The drawing under review shows one solid part. Ordinate dimensions are in mm from its lowest x, y, z. Coordinates: 2 decimals unless noted, no trailing zeros. Order: outer loops, then holes, each group sorted by start corner. A loop starts at its lowest first (then second) coordinate and runs counter-clockwise, first axis right, second up.
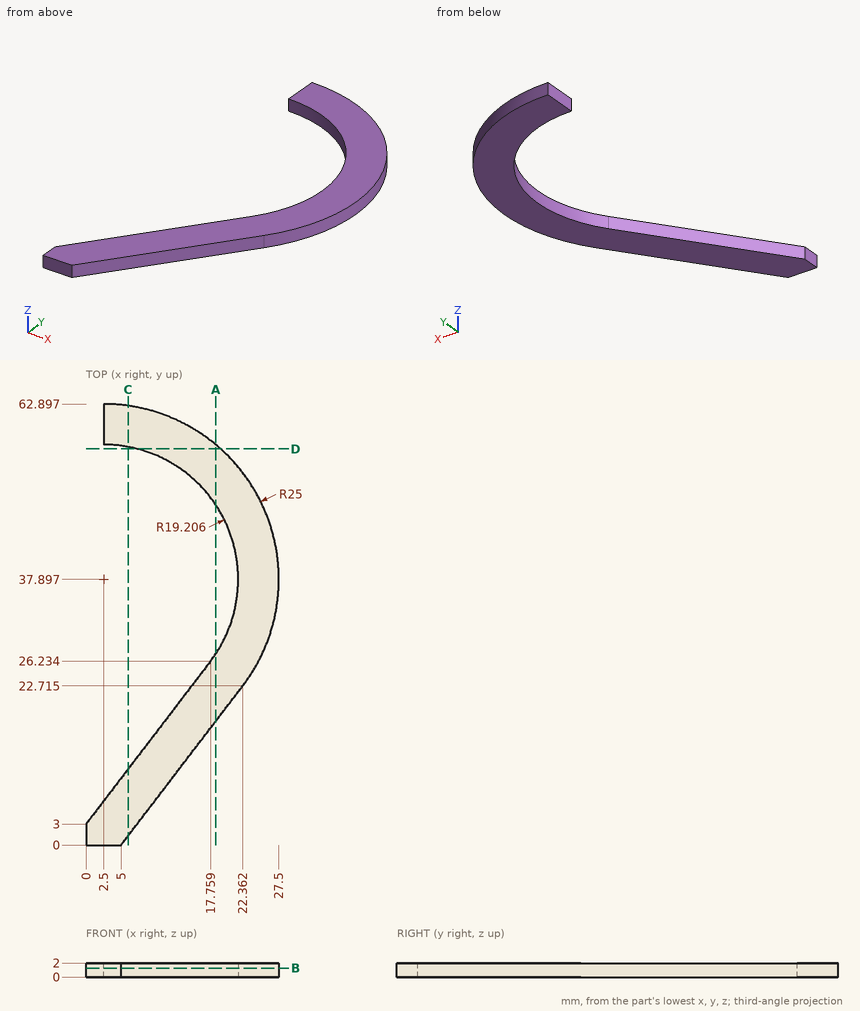
(1) Consider section B-B (z = 1.3). Give the boundary of the cut face in (x, y) (1 decimal), then the cut area to 3 significant figures.
(2) Insertion check: pin 1 Ø0.6 at (y, z) = (60, 0.5) entering from -X. The pin has a flat end and moves straight along its axis. Give the tip position at first contact, or say it passes through.
(3) Consider section D-D (y = 56.5). Give the boundary of the cut face in (x, z) (1 decimal).
(4) Consider section C-C (x = 6). Give the boundary of the cut face in (y, z).
(5) Consider section A-A (x = 18.5). Give the boundary of the cut face in (y, z), then the cut area to 3 significant figures.
(6) Wall thickness on line 1 (X direction, y = 37.5, z = 0.4); line 2 (Y direction, x = 7.5, z = 0.5) (1 decimal); line 3 (Y direction, x = 16, z = 0.55) (1 decimal): over which ranges is each line inside the solid? List them lowest first.
Findings:
1. outline: (0, 0) - (5, 0) - (22.4, 22.7) arc R25 ccw to (2.5, 62.9) - (2.5, 57.1) arc R19.2 cw to (17.8, 26.2) - (0, 3) - close
1. area: 460 mm2
2. pin 1: stops at x = 2.5
3. outline: (7.3, 0) - (19.2, 0) - (19.2, 2) - (7.3, 2) - close
4. outline: (1.31, 0) - (10.85, 0) - (10.85, 2) - (1.31, 2) - close; (56.78, 0) - (62.65, 0) - (62.65, 2) - (56.78, 2) - close
5. outline: (17.66, 0) - (27.27, 0) - (27.27, 2) - (17.66, 2) - close; (48.52, 0) - (57.11, 0) - (57.11, 2) - (48.52, 2) - close
5. area: 36.4 mm2
6. line 1: x = 21.7 to 27.5
6. line 2: y = 3.3 to 12.8, 56.4 to 62.4
6. line 3: y = 14.4 to 23.9, 51.6 to 58.9
